Autodesk Inventor part; units mm, degrees
ref_plane "YZ Plane" through (0, 0, 0) normal (1, 0, 0) x (0, 1, 0)
ref_plane "XZ Plane" through (0, 0, 0) normal (0, 1, 0) x (-1, 0, 0)
ref_plane "XY Plane" through (0, 0, 0) normal (0, 0, 1) x (1, 0, 0)
sketch "Sketch1" plane through (0, 0, 0) normal (0, 1, 0) x (-1, 0, 0)
  circle A0 centre (0, 0) radius 28
  circle A1 centre (0, 0) radius 33
  dimension "d0" = 56
  dimension "d1" = 66
extrude "Extrusion1" add sketch "Sketch1" along normal blind 10
sketch "Sketch2" plane through (0, 10, 0) normal (0, 1, 0) x (1, 0, 0)
  circle A0 centre (0, 0) radius 15
  circle A1 centre (0, 0) radius 33
  dimension "d4" = 30
extrude "Extrusion2" add sketch "Sketch2" along normal blind 5
sketch "Sketch3" plane through (0, 15, 0) normal (0, 1, 0) x (1, 0, 0)
  circle A0 centre (0, 0) radius 15
  circle A1 centre (0, 0) radius 19
  dimension "d7" = 38
  dimension "d8" = 30
extrude "Extrusion3" add sketch "Sketch3" along normal blind 10
properties part number "bigbearingcup" material "Steel"
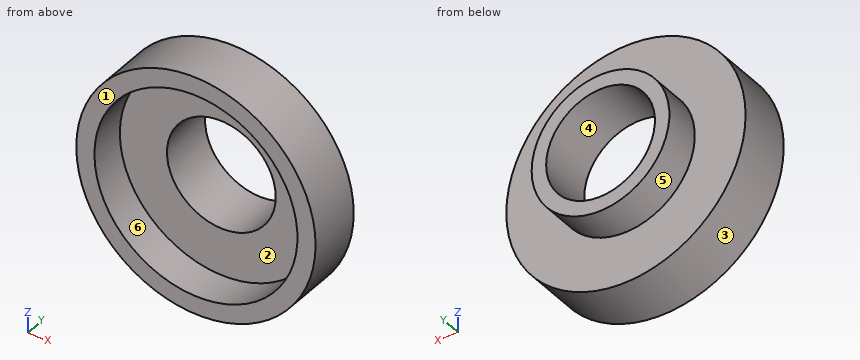
Work out the finished part from the listing and answer in its coordinate system (mm). Face numbers are marked on the shaded views. A direction names the side the tool comes from. Round coordinates to 2 decimals unless told otherwise and drop trailing zeros. Loops run counter-clockwise (first coordinate to the right, second up) from the corner with the lowest first, then second, coordinate; pieces in that order, holes last. Notation, with made-up numbers: M 7.5,77.25 L 23.5,77.25 A22 cw 23.5,107.25 Z; hole C 6.25,32 d7. An arc over 180 degrees is marked long. One line per question, with ' | ' between items.
Q1. A tool of negligible diameter and unlimited length cuts with its end or side. For the marked faces 4, 5 and 6, from which of +Z, -Z, +X, -X, +Y, -Y can it reach the whole face along a straight path? Write none if from no direction.
Conclusion:
face 4: +Y, -Y | face 5: +Y | face 6: -Y
Q2. Consider line 1 along X through (y, z) = (17, -0.5); line 2 along Z through (x, y) = (0, 2); line 3 along X through (y, z) = (13.75, 0). Determine where each line is inside the solid, lowest interval first. Write a range as from..to.
Conclusion:
line 1: x = -18.99..-14.99, 14.99..18.99 | line 2: z = -33..-28, 28..33 | line 3: x = -33..-15, 15..33
Q3. Each of these flat-tipped pins is pushed along its axis until it touches: pin 1 Ø1.5 at (y, z) = (15, -12.5) entering from +X; pin 2 Ø2 at (x, z) = (-18, 24.5) entering from +Y; pin 3 Ø10 at (y, z) = (19.5, 3.5) entering from -X. Where does it stop, or does it pass through?
Conclusion:
pin 1: stops at x = 30.84 | pin 2: stops at y = 15 | pin 3: stops at x = -32.97
Q4. The mould has two halves that part along X. Classify the marked faces 1, 2 and 3: +X half, -X half, draft (parallel to the pull), parting line (faces both ways), or undercut.
Conclusion:
face 1: draft | face 2: undercut | face 3: parting line
Q5. Find section B-B, the plane y = 20. Give the vertices of the cut face in (x, z), then the cut area to 3 significant figures.
Conclusion:
outline: C 0,0 d38; hole C 0,0 d30 | area: 427 mm2
Q6. Find section C-C, the plane y = 11.75. Give the vertices of the cut face in (x, z).
Conclusion:
outline: C 0,0 d66; hole C 0,0 d30
